Can you work these out from the model? Positions are in its coordinate system, mm. Round coordinates to 2 decimals unless told otherwise and drop trailing zeros. Loops run counter-clockwise (first coordinate to the right, second up) from the corner with the lowest first, then second, coordinate; pieces in that order, holes last. Notation, with made-up numbers: M 76.5,-31 L 85.5,-31 A26 ccw 85.5,-2 Z; hole C -6.5,76 d8. An arc over 180 degrees is marked long. Return JSON: item names as keys, results as strings.
Autodesk Fusion 360 part; units mm, degrees
sketch "Sketch1" plane through (0, 0, 0) normal (0, 1, 0) x (1, 0, 0)
  line L0 (0, 0) -> (95, 0)
  line L1 (0, 0) -> (0, 106)
  line L2 (0, 106) -> (95, 106)
  line L3 (95, 106) -> (95, 0)
  line L4 (95, 106) -> (83, 106)
  circle A0 centre (83, 94) radius 7
  line L5 (0, 106) -> (12, 106)
  circle A1 centre (12, 94) radius 7
  circle A2 centre (83, 76) radius 4
  circle A3 centre (12, 76) radius 4
  circle A4 centre (83, 30) radius 4
  circle A5 centre (83, 12) radius 7
  circle A6 centre (12, 30) radius 4
  circle A7 centre (12, 12) radius 7
  circle A8 centre (83, 94) radius 4.25
  circle A9 centre (12, 94) radius 4.25
  circle A10 centre (12, 12) radius 4.25
  circle A11 centre (83, 12) radius 4.25
  dimension "d26" = 8.5
  dimension "d27" = 8.5
  dimension "d28" = 8.5
extrude "Extrude1" add sketch "Sketch1" along normal blind 5 contours L0 L1 L2 L3 L4 L5 | A0 | A1 | A5 | A7
sketch "Sketch2" plane through (0, 5, 0) normal (0, 1, 0) x (-1, 0, 0)
  circle A0 centre (-12, -94) radius 4.25
  circle A1 centre (-83, -76) radius 4
  circle A2 centre (-83, -94) radius 4.25
  circle A3 centre (-12, -76) radius 4
  circle A4 centre (-83, -30) radius 4
  circle A5 centre (-12, -30) radius 4
  circle A6 centre (-83, -12) radius 4.25
  circle A7 centre (-12, -12) radius 4.25
  line L0 (0, 0) -> (-95, 0)
  line L1 (-95, 0) -> (-95, -106)
  line L2 (-95, -106) -> (0, -106)
  line L3 (0, -106) -> (0, 0)
  circle A8 centre (-12, -12) radius 7
  circle A9 centre (-83, -12) radius 7
  circle A10 centre (-83, -94) radius 7
  circle A11 centre (-12, -94) radius 7
  dimension "d31" = 14
  dimension "d32" = 14
  dimension "d33" = 14
  dimension "d34" = 14
extrude "Extrude2" cut sketch "Sketch2" against normal blind 2 contours A8 | A9 | A10 | A11
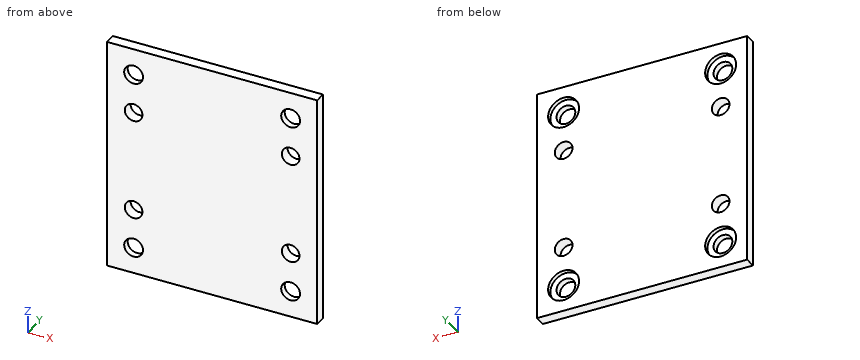
Q1. Suppose I cut it at A-A, the plane z = -12. Please give me the cut outline in (x, y), plus the area to 3 significant figures.
Results:
{"outline": "M 0,0 L 7.75,0 L 7.75,3 L 5,3 L 5,5 L 0,5 Z; M 16.25,0 L 78.75,0 L 78.75,3 L 76,3 L 76,5 L 19,5 L 19,3 L 16.25,3 Z; M 87.25,0 L 95,0 L 95,5 L 90,5 L 90,3 L 87.25,3 Z", "area": "368 mm2"}
Q2. Suppose I cut it at C-C, the plane y = 1.3. State how many separate pieces and enclosed holes the cut face has, plus the area to 3 significant figures.
Results:
{"separate pieces": "1", "enclosed holes": "8", "area": "9,640 mm2"}
Q3. If I drill on line 1 along X through (y, z) = (1.05, -94); line 2 along Z through (x, y) = (83, 4.35); line 3 along Z through (x, y) = (12, 1.2), over which ranges is the centre line in solid material (lowest first)?
Results:
{"line 1": "x = 0 to 7.75, 16.25 to 78.75, 87.25 to 95", "line 2": "z = -106 to -101, -87 to -80, -72 to -34, -26 to -19, -5 to 0", "line 3": "z = -106 to -98.25, -89.75 to -80, -72 to -34, -26 to -16.25, -7.75 to 0"}
Q4. Suppose I cut it at D-D, the plane z = -76. Please give me the cut outline in (x, y), plus the area to 3 significant figures.
Results:
{"outline": "M 0,0 L 8,0 L 8,5 L 0,5 Z; M 16,0 L 79,0 L 79,5 L 16,5 Z; M 87,0 L 95,0 L 95,5 L 87,5 Z", "area": "395 mm2"}
Q5. I'm going to push a flat-ended pin straight in: pin 1 Ø4 at (x, z) = (80, -94.5) entering from +Y. Where does the tip first touch, or does it pass through?
Results:
{"pin 1": "stops at y = 3"}
Q6. Suppose I cut it at B-B, the plane x = 83. Please give me the cut outline in (y, z), plus the area to 3 significant figures.
Results:
{"outline": "M 0,-106 L 5,-106 L 5,-101 L 3,-101 L 3,-98.25 L 0,-98.25 Z; M 0,-89.75 L 3,-89.75 L 3,-87 L 5,-87 L 5,-80 L 0,-80 Z; M 0,-72 L 5,-72 L 5,-34 L 0,-34 Z; M 0,-26 L 5,-26 L 5,-19 L 3,-19 L 3,-16.25 L 0,-16.25 Z; M 0,-7.75 L 3,-7.75 L 3,-5 L 5,-5 L 5,0 L 0,0 Z", "area": "343 mm2"}
